Work out the finished part from the listing and answer in its coordinate system (mm). A direction names the side the tool comes from. Give positions to 0.01 mm unless a question says otherwise; leave off trailing zeros. Write each loop counter-clockwise with the first axis right and the second up, starting at its lowest first coordinate (ties: lowest second). Pieces come first, ordered by that corner, then holes.
1) Straight lines are drawn through the part: probe 1 along X at (y, z) = (-59.25, 17.75); probe 2 along X at (y, z) = (-60.1, 9); probe 3 along Y at (x, z) = (-65, 5.5). For each, find the intervals that lie inside material, in ascending order.
2) Determine the mould class of faces 1 (the face through (-66, -61.366, 12)), 2 (the face through (-63.3, -60.8, 12.3)), 3 (the face through (-66, -60, 25)) for opening direction Y: pulls with the +Y half, pulls with the -Y half, needs draft (parallel to the pull), parting line crosses it, or undercut.
3) Find section B-B (x = -63.25). Determine the outline of the cut face in (y, z), plus the area to 3 significant figures.
4) A tool of negligible diameter and unlimited length cuts with its end or side. For faces 4 (the face through (-66, -60, 0)), 5 (the face through (-69.13, -60.81, 12.32)), from which of +Z, -Z, +X, -X, +Y, -Y can it reach the whole face along a straight path? Write none if from no direction.
5) Given pin 1 Ø1 at (x, y) = (-65, -60.5) entering from -Z, flat-ended and moving along its own axis, determine where the tip first touches the part or whether it passes through.
6) Find section C-C (y = -61.15). Determine the outline of the cut face in (x, z), plus the area to 3 significant figures.
7) Find section A-A (z = 23.5). Determine the outline of the cut face in (x, y).
```python
from build123d import *

# Parameters (mm, degrees)
F1_DEPTH = 25


# Not quite as in the source:
# - ends of sketch curves that miss each other by under 0.0002 mm in the source are joined


with BuildPart() as f1:
    # F0 (on Top) → F1 (new body)
    with BuildSketch(Plane.XY):
        with BuildLine():
            ThreePointArc((-68.7608035324, -59.8356334478), (-68.5298336492, -59.9899625897), (-68.5840268371, -60.2624101431))
            Line((-68.5840268371, -60.2624101431), (-69.6879495324, -61.3663324478))
            Line((-69.6879495324, -61.3663324478), (-62.7336575324, -61.3663328727))
            Line((-62.7336575324, -61.3663328727), (-63.8375805324, -60.2624108727))
            ThreePointArc((-63.8375805324, -60.2624108727), (-63.8917734155, -59.9899625897), (-63.6608035324, -59.8356334478))
            Line((-63.6608035324, -59.8356334478), (-63.4718790681, -59.8356334478))
            Line((-63.4718790681, -59.8356334478), (-63.4718790681, -59.0644426644))
            Line((-63.4718790681, -59.0644426644), (-69.6627650617, -59.0439311215))
            Line((-69.6627650617, -59.0439311215), (-69.6587313915, -59.6062613089))
            Line((-69.6587313915, -59.6062613089), (-69.491799647, -59.8356334478))
            Line((-69.491799647, -59.8356334478), (-68.7608035324, -59.8356334478))
        make_face()
    extrude(amount=F1_DEPTH)


solid = f1.part
```
Results:
1. probe 1: x = -69.66 to -63.47
1. probe 2: x = -68.51 to -63.91
1. probe 3: y = -61.37 to -59.06
2. face 1: pulls with the -Y half
2. face 2: undercut
2. face 3: needs draft
3. outline: (-61.37, 0) - (-60.85, 0) - (-60.85, 25) - (-61.37, 25) - close
3. area: 12.9 mm2
4. face 4: -Z, +X, -X, +Y, -Y
4. face 5: +Z, -Z, -X
5. pin 1: stops at z = 0
6. outline: (-69.47, 0) - (-62.95, 0) - (-62.95, 25) - (-69.47, 25) - close
6. area: 163 mm2
7. outline: (-69.69, -61.37) - (-62.73, -61.37) - (-63.84, -60.26) arc R0.25 cw to (-63.66, -59.84) - (-63.47, -59.84) - (-63.47, -59.06) - (-69.66, -59.04) - (-69.66, -59.61) - (-69.49, -59.84) - (-68.76, -59.84) arc R0.25 cw to (-68.58, -60.26) - close
